Autodesk Inventor part; units mm, degrees
ref_plane "YZ Plane" through (0, 0, 0) normal (1, 0, 0) x (0, 1, 0)
ref_plane "XZ Plane" through (0, 0, 0) normal (0, 1, 0) x (-1, 0, 0)
ref_plane "XY Plane" through (0, 0, 0) normal (0, 0, 1) x (1, 0, 0)
sketch "Sketch1" plane through (0, 0, 0) normal (0, 0, 1) x (1, 0, 0)
  line L0 (0, 0) -> (70, 0)
  line L1 (70, 0) -> (70, 25)
  line L2 (70, 25) -> (15, 25)
  line L3 (15, 25) -> (15, 47.5)
  line L4 (15, 47.5) -> (0, 47.5)
  line L5 (0, 47.5) -> (0, 0)
  point P0 (15, 36.25)
  point P1 (7.5, 47.5)
  dimension "d0" = 15
  dimension "d1" = 25
  dimension "d2" = 47.5
  dimension "d24" = 55
extrude "Extrusion1" add sketch "Sketch1" along normal blind 15
mirror "Mirror1" about plane through (0, 0, 0) normal (0, 1, 0) of "Extrusion1"
sketch "Sketch2" plane through (0, 0, 15) normal (0, 0, 1) x (1, 0, 0)
  circle A0 centre (35, 0) radius 19.75
  line L0 (-14, 0) -> (84, 0)
  line L1 (70, 25) -> (70, -25)
  line L2 (70, 2) -> (35, 2)
  line L3 (35, 2) -> (35, -2)
  line L4 (35, -2) -> (70, -2)
  line L5 (70, -2) -> (70, 2)
  point P0 (0, 0)
  point P1 (52.5, 2)
  point P2 (54.6485, 2)
  point P3 (54.6485, -2)
  dimension "d6" = 39.5
  dimension "d7" = 35
  dimension "d8" = 4
  dimension "d9" = 2
extrude "Extrusion2" cut sketch "Sketch2" against normal through all
sketch "Sketch3" plane through (15, 25, 0) normal (0, 1, 0) x (1, 0, 0)
  line L0 (55, 0) -> (0, 0)
  line L1 (55, 0) -> (55, -15)
  point P0 (-15, 0)
  point P1 (45, -7.5)
  dimension "d12" = 7.5
  dimension "d13" = 10
hole "Hole1" at (60, 25, 7.5) direction (0, -1, 0) diameter 6 end through all
sketch "Sketch4" plane through (15, 25, 0) normal (0, 1, 0) x (1, 0, 0)
  circle A0 centre (45, -7.5) radius 3
  circle A1 centre (45, -7.5) radius 5
  point P0 (-15, 0)
  dimension "d21" = 10
extrude "Extrusion3" cut sketch "Sketch4" against normal blind 15
mirror "Mirror2" about plane through (0, 0, 0) normal (0, 1, 0) of "Extrusion3"
sketch "Sketch5" plane through (15, 25, 0) normal (1, 0, 0) x (0, 0, -1)
  line L0 (0, 0) -> (0, 22.5)
  line L1 (0, 22.5) -> (-15, 22.5)
  point P0 (0, -25)
  point P1 (-7.5, 12.5)
  point P2 (0, 11.25)
  dimension "d26" = 7.5
  dimension "d34" = 10
hole "Hole2" at (15, 37.5, 7.5) direction (-1, 0, 0) diameter 6 end through all
mirror "Mirror3" about plane through (0, 0, 0) normal (0, 1, 0) of "Hole2"
fillet "Fillet1" radius 2 2 edges at (15.25, 0, 15) (15.25, 0, 0)
properties part number "Magazine_Holder_3DPrint"
Read the model definition and answer for the solid it produces. Units are mm, in the model's axes. A direction names the side the tool comes from. Coordinates: 2 decimals unless noted, no trailing zeros. Loops run counter-clockwise (first coordinate to the right, second up) from the corner with the lowest first, then second, coordinate; pieces in that order, holes last. Notation, with made-up numbers: (29.25, 32) -> (47.25, 32) arc R20 ccw to (47.25, 36) -> close; hole circle Ø1 at (71.25, -10.5). An arc over 180 degrees is marked (long way). Return JSON: item names as keys, results as strings.
Item 1: For faces 1 (the flat face through (15, 34, 7)), 2 (the flat face through (58, -10, 10)), 3 (the flat face through (64, 2, 8)), 4 (the flat face through (42, -25, 7)), determine the directions among +Z, -Z, +X, -X, +Y, -Y from which every point of the face is accessible in a straight line to the end or side of a thin tool.
Answers:
{"face 1": "+Z, -Z, +X, +Y", "face 2": "-Y", "face 3": "+Z, -Z, +X", "face 4": "+Z, -Z, +X, -Y"}
Item 2: For a pull along Y with two mould halves and no side action, classify faces 5 (the flat face through (64, -2, 8)), 6 (the cylindrical face through (7.395, 34.526, 7.891)), 7 (the flat face through (62, 10, 10)), 8 (the flat face through (7, -47.5, 7)) as +Y half, -Y half, draft (parallel to the pull), parting line (faces both ways), or undercut.
Answers:
{"face 5": "undercut", "face 6": "undercut", "face 7": "+Y half", "face 8": "-Y half"}
Item 3: Find the intervals of material crossed by probe 1 along Y at (x, z) = (8.25, 7.5); probe 2 along Z at (x, y) = (60, -6); probe 3 along X at (y, z) = (3, 9.25), in increasing order.
Answers:
{"probe 1": "y = -47.5 to -40.5, -34.5 to 34.5, 40.5 to 47.5", "probe 2": "z = 0 to 4.5, 10.5 to 15", "probe 3": "x = 0 to 15.48, 54.52 to 57.56, 62.44 to 70"}
Item 4: Find section C-C (x = 35). Determine the outline of the cut face in (y, z), plus the area to 3 significant figures.
Answers:
{"outline": "(-25, 0) -> (-21.75, 0) arc R2 ccw to (-19.75, 2) -> (-19.75, 13) arc R2 ccw to (-21.75, 15) -> (-25, 15) -> close; (19.75, 2) arc R2 ccw to (21.75, 0) -> (25, 0) -> (25, 15) -> (21.75, 15) arc R2 ccw to (19.75, 13) -> close", "area": "154 mm2"}
Item 5: Find section A-A (x = 60). Determine the outline of the cut face in (y, z), plus the area to 3 significant figures.
Answers:
{"outline": "(-25, 0) -> (-2, 0) -> (-2, 4.5) -> (-10, 4.5) -> (-10, 2.5) -> (-25, 2.5) -> close; (-25, 12.5) -> (-10, 12.5) -> (-10, 10.5) -> (-2, 10.5) -> (-2, 15) -> (-25, 15) -> close; (2, 0) -> (25, 0) -> (25, 2.5) -> (10, 2.5) -> (10, 4.5) -> (2, 4.5) -> close; (2, 10.5) -> (10, 10.5) -> (10, 12.5) -> (25, 12.5) -> (25, 15) -> (2, 15) -> close", "area": "294 mm2"}
Item 6: Find section B-B (y = -37.5). Determine the outline of the cut face in (x, z).
Answers:
{"outline": "(0, 0) -> (15, 0) -> (15, 4.5) -> (0, 4.5) -> close; (0, 10.5) -> (15, 10.5) -> (15, 15) -> (0, 15) -> close"}
Item 7: Flat-ended cylindrical pins translate along their axes: P1, Ø4.5, axis at y = -38.5, z = 7, coming from the +X side; P2, Ø5.5, axis at x = 60, z = 7.5, coming from the +Y side; P3, Ø8, axis at x = 60, z = 7.5, coming from the +Y side; P4, Ø7.5, axis at x = 62.5, z = 10.5, coming from the -Y side. Find the tip coordinate at first contact, or state that the pin passes through.
Answers:
{"P1": "stops at x = 15", "P2": "passes through", "P3": "stops at y = 10", "P4": "stops at y = -25"}
Item 8: Find section D-D (y = -24). Determine the outline of the cut face in (x, z), plus the area to 3 significant figures.
Answers:
{"outline": "(0, 0) -> (70, 0) -> (70, 15) -> (0, 15) -> close; hole circle Ø10 at (60, 7.5)", "area": "971 mm2"}
